Geometry check sheet. Reference: the model listing, model coordinates, mm. A direction names the side the tool comes from. Give positions to 0.01 mm unless a question says otherwise; leave off trailing zeros. Loops run counter-clockwise (first coordinate to the right, second up) from the corner with the lowest first, then second, coordinate; pieces in that order, holes last. Notation, with made-up numbers: (73, -35.75) -> (108, -35.75) arc R34 ccw to (108, -0.75) -> close; hole circle Ø11 at (-26.5, 67). An arc over 180 degrees is marked (long way). One line per item, written item: value. Start each with the question number.
(1) Draft check along X on faces 1 (the face through (-100, -31, 3)), 2 (the face through (100, -31, 3)), 3 (the face through (-65, -1, 3)), 4 (the face through (-94.6, 14.2, 3.4)). Enter one of: pulls with the +X half, pulls with the -X half, needs draft (parallel to the pull), parting line crosses it, or undercut.
(2) Scan lines: line 1 along Y through (x, z) = (-20.5, 2); line 2 along X through (y, z) = (-28, 2.5); line 3 along Y through (x, z) = (44.6, 4). Record each from-to range of solid material in increasing order. Write a range as from..to.
(3) Tool access check on faces 5 (the face through (-1, -23.15, 3)), 6 (the face through (-1, -42.15, 3)). Record the directions out of +Z, -Z, +X, -X, +Y, -Y that give a thin tool (end or side, any length) a straight path to the whole face; none if there is none.
(4) Gauge pin test, flat ends, axial feed: pin 1 Ø8.5 at (x, y) = (92, 16.15) entering from +Z; pin 2 Ø1.5 at (y, z) = (-9.5, 5.5) entering from +X; pin 3 Ø3.5 at (y, z) = (-11, 4.5) entering from +X. Record the tip position at first contact, or that the pin passes through.
(5) Sectioned sample at A-A, the plane x = -1. Record the cut outline in (y, z).
(6) Sectioned sample at D-D, the plane z = 3.75. State how many separate pieces and enclosed holes the cut face has, then the cut area to 3 significant figures.
(7) Sectioned sample at B-B, the plane x = 44.6. Record the cut outline in (y, z), then the cut area to 3 significant figures.
(8) Sectioned sample at C-C, the plane y = -5.5. Record the cut outline in (x, z), then the cut area to 3 significant figures.
from build123d import *

# Parameters (mm, degrees)
SKETCH1_W           = 200
SKETCH1_H           = 84.3
BOSS_EXTRUDE1_DEPTH = 6.8
SKETCH2_R           = 3.25
CUT_EXTRUDE1_DEPTH  = 6.8
FILLET1_R           = 2
SKETCH3_R           = 1.775
SKETCH3_W           = 130
SKETCH3_H           = 44
CUT_EXTRUDE2_DEPTH  = 109.732987175
FILLET2_R           = 2
CUT_EXTRUDE3_DEPTH  = 10
FILLET3_R           = 10


with BuildPart() as part:
    # Sketch1 → Boss-Extrude1 (new body)
    with BuildSketch(Plane.XY):
        Rectangle(SKETCH1_W, SKETCH1_H)
    extrude(amount=BOSS_EXTRUDE1_DEPTH)

    # Sketch2 → Cut-Extrude1 (cut)
    with BuildSketch(Plane.XY.offset(6.8)):
        with Locations((-92, 16.15)):
            Circle(SKETCH2_R)
        with Locations((92, 16.15)):
            Circle(SKETCH2_R)
    extrude(amount=-CUT_EXTRUDE1_DEPTH, mode=Mode.SUBTRACT)

    # Fillet1
    fillet1_edges = [part.edges().sort_by_distance(p)[0] for p in [
        (-100, 42.15, 3.4),
        (100, 42.15, 3.4),
        (100, -42.15, 3.4),
        (-100, -42.15, 3.4),
    ]]
    fillet(fillet1_edges, radius=FILLET1_R)

    # Sketch3 → Cut-Extrude2 (cut, through all)
    with BuildSketch(Plane.XY.offset(6.8)):
        with Locations((-44.6, 26.7722)):
            Circle(SKETCH3_R)
        with Locations((44.6, 26.7722)):
            Circle(SKETCH3_R)
        with Locations((44.6, -29.0722)):
            Circle(SKETCH3_R)
        with Locations((-44.6, -29.0722)):
            Circle(SKETCH3_R)
        with Locations((0, -1.15)):
            Rectangle(SKETCH3_W, SKETCH3_H)
    extrude(amount=-CUT_EXTRUDE2_DEPTH, mode=Mode.SUBTRACT)

    # Fillet2
    fillet2_edges = [part.edges().sort_by_distance(p)[0] for p in [
        (-65, -23.15, 3.4),
        (-65, 20.85, 3.4),
        (65, 20.85, 3.4),
        (65, -23.15, 3.4),
    ]]
    fillet(fillet2_edges, radius=FILLET2_R)

    # Sketch4 → Cut-Extrude3 (cut)
    with BuildSketch(Plane.XY.offset(6.8)):
        with BuildLine():
            Line((-95.764164993, 6.349975114), (-108.891829776, 6.349975114))
            Line((-108.891829776, 6.349975114), (-108.891829776, -12.650024886))
            Line((-108.891829776, -12.650024886), (-95.764164993, -12.650024886))
            ThreePointArc((-95.764164993, -12.650024886), (-86.264164993, -3.150024886), (-95.764164993, 6.349975114))
        make_face()
    cut_extrude3 = extrude(amount=-CUT_EXTRUDE3_DEPTH, mode=Mode.SUBTRACT)

    # Mirror3: Cut-Extrude3 across plane
    add(cut_extrude3.mirror(Plane(origin=(0, 0, 0), x_dir=(0, 0, 1), z_dir=(1, 0, 0))), mode=Mode.SUBTRACT)

    # Fillet3
    fillet3_edges = [part.edges().sort_by_distance(p)[0] for p in [
        (-100, -12.650024886, 3.4),
        (-100, 6.349975114, 3.4),
        (100, 6.349975114, 3.4),
        (100, -12.650024886, 3.4),
    ]]
    fillet(fillet3_edges, radius=FILLET3_R)


solid = part.part
Calculated:
1. face 1: pulls with the -X half
1. face 2: pulls with the +X half
1. face 3: undercut
1. face 4: undercut
2. line 1: y = -42.15..-23.15, 20.85..42.15
2. line 2: x = -100..-46.01, -43.19..43.19, 46.01..100
2. line 3: y = -42.15..-30.85, -27.3..-23.15, 20.85..25, 28.55..42.15
3. face 5: +Z, -Z
3. face 6: +Z, -Z, +X, -X, -Y
4. pin 1: stops at z = 6.8
4. pin 2: stops at x = 89.45
4. pin 3: stops at x = 94.3
5. outline: (-42.15, 0) -> (-23.15, 0) -> (-23.15, 6.8) -> (-42.15, 6.8) -> close; (20.85, 0) -> (42.15, 0) -> (42.15, 6.8) -> (20.85, 6.8) -> close
6. separate pieces: 1
6. enclosed holes: 7
6. area: 10,500 mm2
7. outline: (-42.15, 0) -> (-30.85, 0) -> (-30.85, 6.8) -> (-42.15, 6.8) -> close; (-27.3, 0) -> (-23.15, 0) -> (-23.15, 6.8) -> (-27.3, 6.8) -> close; (20.85, 0) -> (25, 0) -> (25, 6.8) -> (20.85, 6.8) -> close; (28.55, 0) -> (42.15, 0) -> (42.15, 6.8) -> (28.55, 6.8) -> close
7. area: 226 mm2
8. outline: (-86.56, 0) -> (-65, 0) -> (-65, 6.8) -> (-86.56, 6.8) -> close; (65, 0) -> (86.56, 0) -> (86.56, 6.8) -> (65, 6.8) -> close
8. area: 293 mm2
